The listing builds one solid part. Answer for the finished solid, in the listing's coordinates (mm). A direction names the side the tool comes from. Coordinates: 2 decimals unless noted, no trailing zeros. Loops run counter-clockwise (first coordinate to the right, second up) from the corner with the lowest first, then second, coordinate; pieces in that order, holes last. Notation, with made-up numbers: (-20, 44.5) - (39, 44.5) arc R14 ccw to (39, 64.5) - close; hole circle Ø1 at (86, 9). An arc over 180 degrees is marked (long way). Return JSON: item names as keys, results as strings. Group by question number.
1. Section A-A (y = 18.5) is taken. Write down the section's boundary in (x, z) (3 decimals), and give its area (3 significant figures).
2. The mould has two halves that part along Y. Classify faces 4 (the face through (0.167, 15.724, -0.144)), 5 (the face through (0, 31.7, 0)), 6 (the face through (-1.686, 1.014, 2.976)), 7 (the face through (0, 0, 2)): pulls with the +Y half, pulls with the -Y half, needs draft (parallel to the pull), parting line crosses it, or undercut.
3. Find the intervals of material crossed by line 1 along Y through (x, z) = (1.75, 1.25); line 2 along Z through (x, y) = (0, 4.5); line 3 along Y through (x, z) = (-0.5, -2.5), in increasing order.
4. Each of these flat-tipped pins is pushed along its axis until it touches: P1, Ø1.6, axis at y = 1, z = 0.5, coming from the +X side; P2, Ø1.5, axis at y = 16, z = 1.5, coming from the +X side; P3, Ø3, axis at x = -3, y = 8.5, coming from the -Z side; P4, Ø1, axis at y = 24.5, z = 3.5, coming from the +X side. Where does it stop, or does it pass through?
5. Which of the six approach directions +Z, -Z, +X, -X, +Y, -Y give full straight-line access (tool end or side, diameter ignored) to faces 1 (the face through (2, 2, -3)), 2 (the face through (1.73, 1.01, 2.95)), 3 (the face through (3.421, 1, 0))?
```python
from build123d import *

# Parameters (mm, degrees)
TAGLIO_ESTRUSIONE1_START      = -2
SCHIZZO2_R                    = 4.5
TAGLIO_ESTRUSIONE1_DEPTH      = 2
FORO_FILETTATO_M3X0_5_1_D     = 2.5
FORO_FILETTATO_M3X0_5_1_DEPTH = 9
FORO_FILETTATO_M3X0_5_1_TIP   = 0.751075774
SCHIZZO5_R                    = 1
TAGLIO_ESTRUSIONE2_DEPTH      = 34.021984674


with BuildPart() as part:
    # Schizzo1 → Rivoluzione1 (revolve)
    with BuildSketch(Plane.XY, mode=Mode.PRIVATE) as rivoluzione1_sk:
        with BuildLine():
            Line((0, 0), (4.5, 0))
            Line((4.5, 0), (4.5, 6.215934246))
            ThreePointArc((4.5, 6.215934246), (4.461941718, 6.489188945), (4.350663738, 6.741644436))
            Line((4.350663738, 6.741644436), (3.104336262, 8.758355564))
            ThreePointArc((3.104336262, 8.758355564), (2.993058282, 9.010811055), (2.955, 9.284065754))
            Line((2.955, 9.284065754), (2.955, 31.7))
            Line((2.955, 31.7), (0, 31.7))
            Line((0, 31.7), (0, 0))
        make_face()
    revolve(rivoluzione1_sk.sketch.rotate(Axis((0, 31.7, 0), (0, -1, 0)), 180), axis=Axis((0, 31.7, 0), (0, -1, 0)))

    # Schizzo2 → Taglio-Estrusione1 (cut)
    with BuildSketch(Plane.XZ.offset(TAGLIO_ESTRUSIONE1_START)):
        with Locations(Location((0, 0, 0), (0, 0, 180))):
            Circle(SCHIZZO2_R)
        Polygon((0, 3.95), (-3.420800345, 1.975), (-3.420800345, -1.975), (0, -3.95), (3.420800345, -1.975), (3.420800345, 1.975), align=None, mode=Mode.SUBTRACT)
    extrude(amount=TAGLIO_ESTRUSIONE1_DEPTH, mode=Mode.SUBTRACT)

    # Foro filettato M3x0.5-1
    with Locations(Plane(origin=(0, 0, 0), x_dir=(-1, 0, 0), z_dir=(0, -1, 0))):
        with Locations((0, 0)):
            Hole(FORO_FILETTATO_M3X0_5_1_D / 2, depth=FORO_FILETTATO_M3X0_5_1_DEPTH)
            with Locations((0, 0, -(FORO_FILETTATO_M3X0_5_1_DEPTH + FORO_FILETTATO_M3X0_5_1_TIP / 2))):  # 118° drill point
                Cone(0, FORO_FILETTATO_M3X0_5_1_D / 2, FORO_FILETTATO_M3X0_5_1_TIP, mode=Mode.SUBTRACT)

    # Schizzo5 → Taglio-Estrusione2 (cut, through all)
    with BuildSketch(Plane(origin=(-1.4775, 0, -2.559105068), x_dir=(-0.8660254037844385, 0, 0.5000000000000004), z_dir=(-0.5000000000000003, 0, -0.8660254037844384))):
        with Locations((0, 16.7)):
            Circle(SCHIZZO5_R)
        with Locations((0, 20.7)):
            Circle(SCHIZZO5_R)
        with Locations((0, 24.7)):
            Circle(SCHIZZO5_R)
        with Locations((0, 28.7)):
            Circle(SCHIZZO5_R)
    extrude(amount=-TAGLIO_ESTRUSIONE2_DEPTH, mode=Mode.SUBTRACT)


solid = part.part
```
The answers:
{
 "1": {"outline": "circle Ø5.91 at (0, 0)", "area": "27.4 mm2"},
 "2": {"face 4": "undercut", "face 5": "pulls with the +Y half", "face 6": "needs draft", "face 7": "pulls with the -Y half"},
 "3": {"line 1": "y = 0 to 16.25, 17.15 to 20.25, 21.15 to 24.25, 25.15 to 28.25, 29.15 to 31.7", "line 2": "z = -4.5 to -1.25, 1.25 to 4.5", "line 3": "y = 0 to 16.12, 17.28 to 20.12, 21.28 to 24.12, 25.28 to 28.12, 29.28 to 31.7"},
 "4": {"P1": "stops at x = 3.42", "P2": "stops at x = 2.86", "P3": "stops at z = -3.41", "P4": "passes through"},
 "5": {"face 1": "-Y", "face 2": "+Z, +X, -Y", "face 3": "+Z, -Z, +X, -Y"}
}
